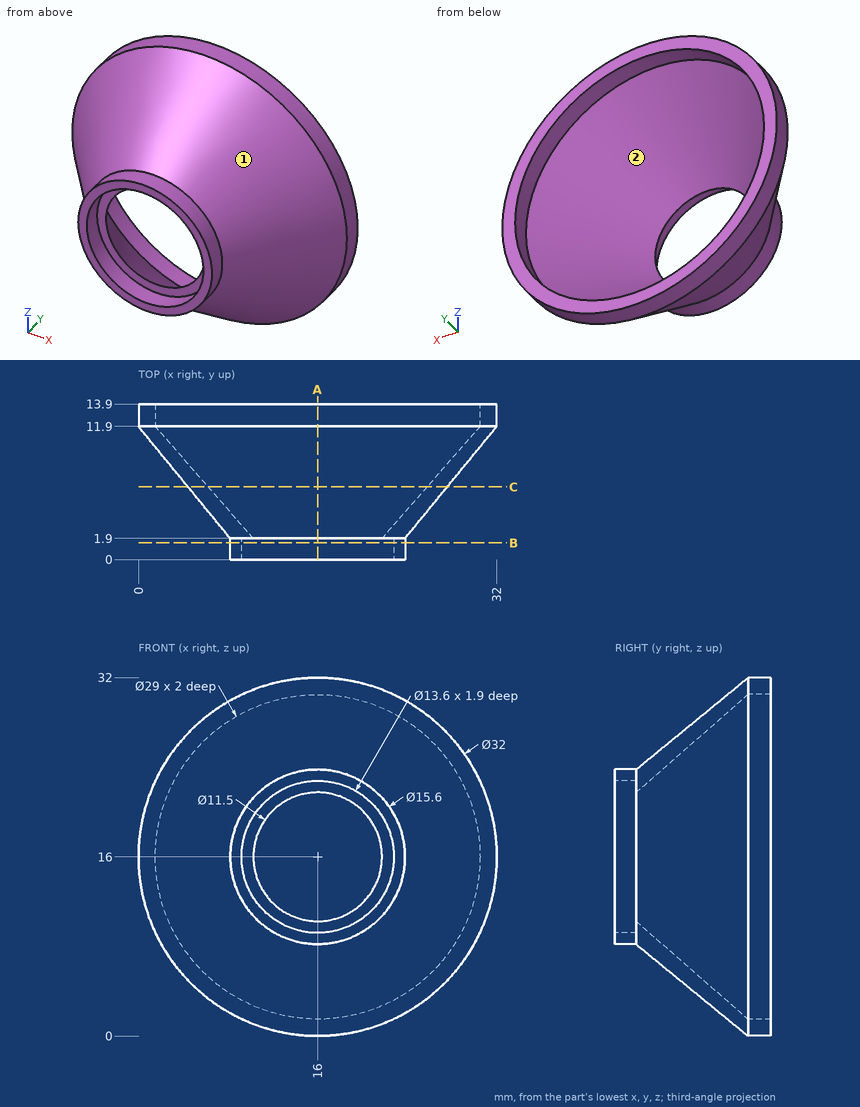
Source: three-view drawing plus pictorial views. Frame: mm from the lowest corner of the part. Coordinates: 2 decimals unless noted, no trailing zeros. Order: outer loops, then holes, each group sorted by start corner. A loop starts at its lowest first (then second) coordinate and runs counter-clockwise, first axis right, second up. Notation, with made-up numbers: (-25.5, 77) -> (20.5, 77) arc R21 cw to (20.5, 92) -> close; hole circle Ø3 at (-11.5, -34.5). An arc over 180 degrees is marked (long way). Write item = value, one per line.
(1) Cut plane B-B on y = 1.5. Return loops of the section in (x, z).
Solved:
outline = circle Ø15.6 at (16, 16); hole circle Ø13.6 at (16, 16)
(2) Line query: line 1 (Z direction, x = 16, y = 1.35); line 2 (Z direction, x = 16, y = 13.3); line 3 (X direction, y = 11, z = 17). Output: solid intervals per line, ascending.
Solved:
line_1 = 8.2 to 9.2, 22.8 to 23.8
line_2 = 0 to 1.5, 30.5 to 32
line_3 = 0.77 to 2.32, 29.68 to 31.23
(3) Pin query (flat end, axial travel): pin 1 Ø3 at (x, y) = (16.5, 11.5) entering from +Z; pin 2 Ø1.5 at (y, z) = (12, 28.5) entering from -X; pin 3 Ø1.5 at (y, z) = (4.5, 9) entering from +X; pin 4 Ø4 at (y, z) = (7, 9) entering from +X. Return the tip coordinate at first contact, or that it passes through.
Solved:
pin_1 = 32
pin_2 = 5.14
pin_3 = 24.11
pin_4 = 27.98
(4) Pull-direction query (Z, two-part tool) for the marked faces 1 and 2; classes: pulls with the +Z half, pulls with the -Z half, needs draft (parallel to the pull), parting line crosses it, or undercut.
Solved:
face_1 = parting line crosses it
face_2 = undercut
(5) Cut plane A-A on x = 16. Return loops of the section in (y, z), plus the area to 3 significant figures.
Solved:
outline = (0, 8.2) -> (1.9, 8.2) -> (11.9, 0) -> (13.9, 0) -> (13.9, 1.5) -> (11.9, 1.5) -> (1.9, 10.25) -> (1.9, 9.2) -> (0, 9.2) -> close; (0, 22.8) -> (1.9, 22.8) -> (1.9, 21.75) -> (11.9, 30.5) -> (13.9, 30.5) -> (13.9, 32) -> (11.9, 32) -> (1.9, 23.8) -> (0, 23.8) -> close
area = 45.3 mm²
(6) Cut plane C-C on y = 6.5. Return loops of the section in (x, z) (3 decimals).
Solved:
outline = circle Ø23.144 at (16, 16); hole circle Ø19.55 at (16, 16)
